Can you work these out from the model? Positions are in its coordinate system, mm. A direction names the side the tool comes from. Coordinates: 2 decimals unless noted, no trailing zeros. Order: outer loops, then holes, each group sorted by start corner. A loop starts at its lowest first (then second) coordinate and runs counter-clockwise, first axis right, second up.
```python
from build123d import *

# Parameters (mm, degrees)
BOSS_EXTRUDE1_DEPTH = 17
SKETCH17_W          = 17
SKETCH17_H          = 17
BOSS_EXTRUDE2_DEPTH = 3
CUT_EXTRUDE1_DEPTH  = 13
SKETCH23_W          = 17
SKETCH23_H          = 20
BOSS_EXTRUDE3_DEPTH = 3
SKETCH24_W          = 12
SKETCH24_H          = 1
CUT_EXTRUDE2_DEPTH  = 3
CUT_EXTRUDE3_REACH  = 29.591
SKETCH30_W          = 12
SKETCH30_H          = 1
CUT_EXTRUDE4_DEPTH  = 28.590759323
CUT_EXTRUDE5_DEPTH  = 28.590759323
SKETCH39_W          = 12
SKETCH39_H          = 3
CUT_EXTRUDE6_DEPTH  = 1
SKETCH40_W          = 6
SKETCH40_H          = 1
BOSS_EXTRUDE4_DEPTH = 2.5
SKETCH41_W          = 6
SKETCH41_H          = 1
BOSS_EXTRUDE5_DEPTH = 2.5
BOSS_EXTRUDE6_REACH = 32.57
SKETCH49_W          = 6
SKETCH49_H          = 1
SKETCH50_W          = 12
SKETCH50_H          = 3
CUT_EXTRUDE7_DEPTH  = 1
SKETCH51_W          = 6
SKETCH51_H          = 1
BOSS_EXTRUDE7_DEPTH = 2.5
FILLET1_R           = 0.5


with BuildPart() as part:
    # Sketch16 → Boss-Extrude1 (new body)
    with BuildSketch(Plane(origin=(8.5, 0, 0), x_dir=(0, 0, -1), z_dir=(1, 0, 0))):
        Polygon((-3, 3), (-3, 20), (-20, 3), align=None)
    extrude(amount=-BOSS_EXTRUDE1_DEPTH)

    # Sketch17 → Boss-Extrude2 (add)
    with BuildSketch(Plane(origin=(0, 0, 3), x_dir=(-1, 0, 0), z_dir=(0, 0, -1))):
        with Locations((0, 11.5)):
            Rectangle(SKETCH17_W, SKETCH17_H)
    extrude(amount=BOSS_EXTRUDE2_DEPTH)

    # Sketch22 → Cut-Extrude1 (cut)
    with BuildSketch(Plane(origin=(6.5, 0, 0), x_dir=(0, 0, -1), z_dir=(1, 0, 0))):
        Polygon((-3, 20), (-20, 3), (-3, 3), align=None)
    extrude(amount=-CUT_EXTRUDE1_DEPTH, mode=Mode.SUBTRACT)

    # Sketch23 → Boss-Extrude3 (add)
    with BuildSketch(Plane.XZ.offset(-3)):
        with Locations((0, 10)):
            Rectangle(SKETCH23_W, SKETCH23_H)
    extrude(amount=BOSS_EXTRUDE3_DEPTH)

    # Sketch24 → Cut-Extrude2 (cut)
    with BuildSketch(Plane.XZ):
        with Locations((0, 0.5)):
            Rectangle(SKETCH24_W, SKETCH24_H)
    extrude(amount=-CUT_EXTRUDE2_DEPTH, mode=Mode.SUBTRACT)

    # Sketch30 → Cut-Extrude3 (cut, up to next)
    with BuildSketch(Plane.XY.offset(3), mode=Mode.PRIVATE) as cut_extrude3_sk1:
        with Locations((0, 0.5)):
            Rectangle(SKETCH30_W, SKETCH30_H)
    cut_extrude3_tool1 = extrude(cut_extrude3_sk1.sketch, amount=-CUT_EXTRUDE3_REACH, mode=Mode.PRIVATE) & part.part
    add(cut_extrude3_tool1.solids().sort_by_distance((0, 0.5, 3))[0], mode=Mode.SUBTRACT)

    # Sketch37 → Cut-Extrude4 (cut, through all)
    with BuildSketch(Plane.XY.offset(3)):
        with BuildLine():
            Line((2.75, 8), (2.75, 13))
            ThreePointArc((2.75, 13), (0, 15.75), (-2.75, 13))
            Line((-2.75, 13), (-2.75, 8))
            ThreePointArc((-2.75, 8), (0, 5.25), (2.75, 8))
        make_face()
    extrude(amount=-CUT_EXTRUDE4_DEPTH, mode=Mode.SUBTRACT)

    # Sketch38 → Cut-Extrude5 (cut, through all)
    with BuildSketch(Plane(origin=(0, 3, 0), x_dir=(-1, 0, 0), z_dir=(0, 1, 0))):
        with BuildLine():
            Line((-2.75, 13), (-2.75, 8))
            ThreePointArc((-2.75, 8), (0, 5.25), (2.75, 8))
            Line((2.75, 8), (2.75, 13))
            ThreePointArc((2.75, 13), (0, 15.75), (-2.75, 13))
        make_face()
    extrude(amount=-CUT_EXTRUDE5_DEPTH, mode=Mode.SUBTRACT)

    # Sketch39 → Cut-Extrude6 (cut)
    with BuildSketch(Plane.XZ):
        with Locations((0, 17.5)):
            Rectangle(SKETCH39_W, SKETCH39_H)
    extrude(amount=-CUT_EXTRUDE6_DEPTH, mode=Mode.SUBTRACT)

    # Sketch40 → Boss-Extrude4 (add)
    with BuildSketch(Plane.XZ.offset(-1)):
        with Locations((0, 17.5)):
            Rectangle(SKETCH40_W, SKETCH40_H)
    extrude(amount=BOSS_EXTRUDE4_DEPTH)

    # Sketch41 → Boss-Extrude5 (add)
    with BuildSketch(Plane.XZ.offset(-1)):
        with Locations((0, 1.5)):
            Rectangle(SKETCH41_W, SKETCH41_H)
    extrude(amount=BOSS_EXTRUDE5_DEPTH)

    # Sketch49 → Boss-Extrude6 (add, up to next)
    with BuildSketch(Plane(origin=(0, 0, -1.5), x_dir=(-1, 0, 0), z_dir=(0, 0, -1)), mode=Mode.PRIVATE) as boss_extrude6_sk1:
        with Locations((0, 1.5)):
            Rectangle(SKETCH49_W, SKETCH49_H)
    boss_extrude6_tool1 = extrude(boss_extrude6_sk1.sketch, amount=-BOSS_EXTRUDE6_REACH, mode=Mode.PRIVATE) - part.part
    add(boss_extrude6_tool1.solids().sort_by_distance((0, 1.5, -1.5))[0])

    # Sketch50 → Cut-Extrude7 (cut)
    with BuildSketch(Plane(origin=(0, 0, 0), x_dir=(-1, 0, 0), z_dir=(0, 0, -1))):
        with Locations((0, 17.5)):
            Rectangle(SKETCH50_W, SKETCH50_H)
    extrude(amount=-CUT_EXTRUDE7_DEPTH, mode=Mode.SUBTRACT)

    # Sketch51 → Boss-Extrude7 (add)
    with BuildSketch(Plane(origin=(0, 0, 1), x_dir=(-1, 0, 0), z_dir=(0, 0, -1))):
        with Locations((0, 17.5)):
            Rectangle(SKETCH51_W, SKETCH51_H)
    extrude(amount=BOSS_EXTRUDE7_DEPTH)

    # Fillet1
    fillet1_edges = [part.edges().sort_by_distance(p)[0] for p in [
        (0, 3, 3),
    ]]
    fillet(fillet1_edges, radius=FILLET1_R)


solid = part.part
```
1. Thinking about a two-plate mould opening in X: for faces 1 (the flat face through (0, 17.5, -1.5)), 2 (the flat face through (-3, -0.2, 17.5)), 3 (the flat face through (-8.5, 8, 8)), which applies, pulls with the +X half, pulls with the -X half, needs draft (parallel to the pull), parting line crosses it, or undercut?
Completed:
face 1: needs draft
face 2: undercut
face 3: pulls with the -X half
2. Please list where these lines run through material, in increasing order: probe 1 along X at (y, z) = (16, 4.75); probe 2 along Y at (x, z) = (4, 8.75); probe 3 along Y at (x, z) = (-5.25, 17.75).
Completed:
probe 1: x = -8.5 to -6.5, 6.5 to 8.5
probe 2: y = 0 to 3
probe 3: y = 1 to 3
3. Imagine slicing it at D-D on x = 0. Give the number of separate pieces and of enclosed holes in the cut face, then the cut area to 3 significant figures.
Completed:
separate pieces: 3
enclosed holes: 0
area: 47.1 mm2
4. Imagine slicing it at C-C on x = 3.75. Please give me the cut outline in (y, z), then the cut area to 3 significant figures.
Completed:
outline: (0, 3) - (1, 3) - (1, 1) - (3, 1) - (3, 0) - (16, 0) - (16, 1) - (19, 1) - (19, 0) - (20, 0) - (20, 3) - (3.5, 3) arc R0.5 cw to (3, 3.5) - (3, 20) - (0, 20) - (0, 19) - (1, 19) - (1, 16) - (0, 16) - close
area: 100 mm2
5. I'm going to push flat-ended pins straight in: pin 1 (5 mm diameter, centred on x = -3, y = 5.5, fed in from -Z); pin 2 (0.8 mm diameter, centred on x = -0.5, y = 0.5, fed in from -Z); pin 3 (0.5 mm diameter, centred on x = 2.5, z = 0.5, fed in from -Y). Where does each tip first touch, or does it pass through?
Completed:
pin 1: stops at z = 0
pin 2: stops at z = 1
pin 3: stops at y = 1
6. Imagine slicing it at B-B on z = 6.25. Please give me the cut outline in (x, y).
Completed:
outline: (-8.5, 0) - (-2.12, 0) - (-2.12, 3) - (-6.5, 3) - (-6.5, 16.75) - (-8.5, 16.75) - close; (2.12, 0) - (8.5, 0) - (8.5, 16.75) - (6.5, 16.75) - (6.5, 3) - (2.12, 3) - close
7. On a 3-axis mill with a long thin cutter (end or side, diameter ignored), from which of +Z, -Z, +X, -X, +Y, -Y can I reach the whole of each face in a straight line? I mean faces 4 (the flat face through (-3, -0.2, 1.5)), 5 (the flat face through (6.5, 8, 8)), 6 (the flat face through (-6, 0.5, 17.5)), 7 (the flat face through (2.75, 10, 2)), 8 (the flat face through (0, 18, 0)). Say none if no direction works.
Completed:
face 4: -Z, -Y
face 5: +Z, +Y
face 6: -Y
face 7: +Z, -Z
face 8: -Z
8. Imagine slicing it at A-A on y = 12. Please give me the cut outline in (x, z).
Completed:
outline: (-8.5, 0) - (-2.75, 0) - (-2.75, 3) - (-6.5, 3) - (-6.5, 11) - (-8.5, 11) - close; (2.75, 0) - (8.5, 0) - (8.5, 11) - (6.5, 11) - (6.5, 3) - (2.75, 3) - close
